Here's how the part is built. I have some questions about the finished solid (model axes, mm). A direction names the side the tool comes from. Give positions to 0.01 mm unless a question says otherwise; leave off trailing zeros. Loops run counter-clockwise (first coordinate to the right, second up) from the corner with the lowest first, then second, coordinate; pieces in that order, holes last.
Q1. For faces 4 (the face through (0.493, -40.669, 17.255)), 5 (the face through (47, -17, 15)), 6 (the face through (3, -39, 19)), 7 (the face through (45, -17, 31)), which set-ups out of +Z, -Z, +X, -X, +Y, -Y let a thin tool reach every point of the face, with its end or its side?
Q2. If we section it at C-C (y = -29.5): Please give me the cut outline in (x, z), plus the area to 3 significant figures.
Q3. We'd pull the mould along Y, two halves only. Please class faces 1 (the face through (1.5, -41, 7.6)), 2 (the face through (51.255, -0.493, 22.269)), 3 (the face through (6, -17, 31)): +Y half, -Y half, draft (parallel to the pull), parting line (faces both ways), or undercut.
Q4. If we section it at B-B (x = 31): Please give me the cut outline in (y, z).
Q5. Will these pins go through, and if not, where does the flat tip stop? P1, Ø5, axis at y = -41.5, z = 20.5, coming from the -X side; P2, Ø1.5, axis at x = 12, z = 11.5, coming from the -Y side; P3, Ø13.5, axis at y = -21.5, z = 21.5, coming from the +X side.
Q6. If we section it at D-D (z = 11): Please give me the cut outline in (x, y), plus the area to 3 significant figures.
Q7. I need wall thicknesses on line 1 (Y direction, x = 37, z = 9); line 2 (X direction, y = -18.5, z = 26.5); line 3 (Y direction, x = 61, z = 14). Which ranges of each line are inside material? Lowest first, please.
Q8. If we section it at A-A (z = 22.5): Please give me the cut outline in (x, y).
from build123d import *

# Parameters (mm, degrees)
ESBO_O1_W                = 39
ESBO_O1_H                = 27.4
RESSALTO_EXTRUS_O1_DEPTH = 32
ESBO_O2_W                = 43
ESBO_O2_H                = 27.4
CORTE_EXTRUS_O1_DEPTH    = 30
ESBO_O3_R                = 1.75
CORTE_EXTRUS_O2_DEPTH    = 6
ESBO_O4_R                = 1.75
CORTE_EXTRUS_O3_DEPTH    = 6
CHANFRO1_SIZE            = 15
ESBO_O5_R                = 5.25
CORTE_EXTRUS_O4_DEPTH    = 1
ESBO_O6_R                = 5.25
CORTE_EXTRUS_O5_DEPTH    = 1


with BuildPart() as part:
    # Esboço1 → Ressalto-extrusão1 (new body)
    with BuildSketch(Plane.XY):
        Polygon((0, 0), (64, 0), (64, -3), (49, -3), (49, -33.4), (3, -33.4), (3, -48.4), (0, -48.4), align=None)
        with Locations((25.5, -16.7)):
            Rectangle(ESBO_O1_W, ESBO_O1_H, mode=Mode.SUBTRACT)
    extrude(amount=RESSALTO_EXTRUS_O1_DEPTH)

    # Esboço2 → Corte-extrusão1 (cut)
    with BuildSketch(Plane(origin=(0, 0, 0), x_dir=(-1, 0, 0), z_dir=(0, 0, -1))):
        with Locations((-25.5, -16.7)):
            Rectangle(ESBO_O2_W, ESBO_O2_H)
    extrude(amount=-CORTE_EXTRUS_O1_DEPTH, mode=Mode.SUBTRACT)

    # Esboço3 → Corte-extrusão2 (cut)
    with BuildSketch(Plane.XZ.offset(3)):
        with Locations((56.5, 22.5)):
            Circle(ESBO_O3_R)
    extrude(amount=-CORTE_EXTRUS_O2_DEPTH, mode=Mode.SUBTRACT)

    # Esboço4 → Corte-extrusão3 (cut)
    with BuildSketch(Plane(origin=(3, 0, 0), x_dir=(0, 0, -1), z_dir=(1, 0, 0))):
        with Locations((-22.5, -40.9)):
            Circle(ESBO_O4_R)
    extrude(amount=-CORTE_EXTRUS_O3_DEPTH, mode=Mode.SUBTRACT)

    # Chanfro1
    chanfro1_edges = [part.edges().sort_by_distance(p)[0] for p in [
        (1.5, -48.4, 0),
        (64, -1.5, 0),
    ]]
    chamfer(chanfro1_edges, length=CHANFRO1_SIZE)

    # Esboço5 → Corte-extrusão4 (cut)
    with BuildSketch(Plane(origin=(0, 0, 0), x_dir=(1, 0, 0), z_dir=(0, 1, 0))):
        with Locations((56.5, -22.5)):
            Circle(ESBO_O5_R)
    extrude(amount=-CORTE_EXTRUS_O4_DEPTH, mode=Mode.SUBTRACT)

    # Esboço6 → Corte-extrusão5 (cut)
    with BuildSketch(Plane.ZY):
        with Locations((22.5, -40.9)):
            Circle(ESBO_O6_R)
    extrude(amount=-CORTE_EXTRUS_O5_DEPTH, mode=Mode.SUBTRACT)


solid = part.part
Check sheet entries:
1. face 4: -X
1. face 5: -Z
1. face 6: +Z, -Z, +X, -Y
1. face 7: +Z, -Z
2. outline: (0, 0) - (4, 0) - (4, 30) - (6, 30) - (6, 32) - (0, 32) - close; (45, 30) - (47, 30) - (47, 0) - (49, 0) - (49, 32) - (45, 32) - close
2. area: 200 mm2
3. face 1: -Y half
3. face 2: draft
3. face 3: undercut
4. outline: (-33.4, 0) - (-30.4, 0) - (-30.4, 32) - (-33.4, 32) - close; (-3, 0) - (0, 0) - (0, 32) - (-3, 32) - close
5. P1: stops at x = 1
5. P2: stops at y = -33.4
5. P3: stops at x = 49
6. outline: (0, -44.4) - (3, -44.4) - (3, -33.4) - (49, -33.4) - (49, -3) - (60, -3) - (60, 0) - (0, 0) - close; hole (4, -30.4) - (47, -30.4) - (47, -3) - (4, -3) - close
6. area: 524 mm2
7. line 1: y = -33.4 to -30.4, -3 to 0
7. line 2: x = 0 to 4, 47 to 49
7. line 3: y = -3 to 0
8. outline: (0, -48.4) - (3, -48.4) - (3, -42.65) - (1, -42.65) - (1, -46.15) - (0, -46.15) - close; (0, -35.65) - (1, -35.65) - (1, -39.15) - (3, -39.15) - (3, -33.4) - (49, -33.4) - (49, -3) - (54.75, -3) - (54.75, -1) - (51.25, -1) - (51.25, 0) - (0, 0) - close; (58.25, -3) - (64, -3) - (64, 0) - (61.75, 0) - (61.75, -1) - (58.25, -1) - close; hole (4, -30.4) - (47, -30.4) - (47, -3) - (4, -3) - close
